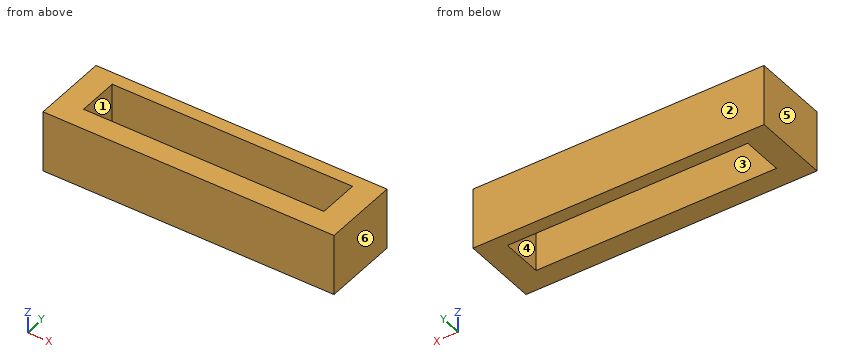
Autodesk Inventor part; units mm, degrees
ref_plane "YZ Plane" through (0, 0, 0) normal (1, 0, 0) x (0, 1, 0)
ref_plane "XZ Plane" through (0, 0, 0) normal (0, 1, 0) x (-1, 0, 0)
ref_plane "XY Plane" through (0, 0, 0) normal (0, 0, 1) x (1, 0, 0)
sketch "Sketch1" plane through (0, 0, 0) normal (0, 1, 0) x (-1, 0, 0)
  line L0 (-19.3909, 30.3636) -> (13.9091, 30.3636)
  line L1 (13.9091, 30.3636) -> (13.9091, 37.3636)
  line L2 (13.9091, 37.3636) -> (-19.3909, 37.3636)
  line L3 (-19.3909, 37.3636) -> (-19.3909, 30.3636)
  point P0 (0, 0)
  dimension "d0" = 33.3
  dimension "d1" = 7
extrude "MainBody" add sketch "Sketch1" along normal blind 2.5
sketch "Sketch2" plane through (0, 2.5, 0) normal (0, 1, 0) x (1, 0, 0)
  line L0 (-13.9091, -30.3636) -> (-13.9091, -37.3636)
  line L1 (-13.9091, -30.3636) -> (-11.0091, -30.3636)
  line L2 (-11.0091, -30.3636) -> (-11.0091, -37.3636)
  line L3 (-11.0091, -37.3636) -> (-13.9091, -37.3636)
  line L4 (-13.9091, -37.3636) -> (-13.9091, -30.3636)
  line L5 (-13.9091, -37.3636) -> (19.3909, -37.3636)
  line L6 (19.3909, -37.3636) -> (19.3909, -30.3636)
  line L7 (16.4909, -37.3636) -> (19.3909, -37.3636)
  line L8 (19.3909, -37.3636) -> (19.3909, -30.3636)
  line L9 (19.3909, -30.3636) -> (16.4909, -30.3636)
  line L10 (16.4909, -30.3636) -> (16.4909, -37.3636)
  line L11 (19.3909, -30.3636) -> (-13.9091, -30.3636)
  point P0 (0, 0)
  point P1 (-13.9091, -37.3636)
  dimension "ClipWidth" = 2.9
  dimension "d5" = 7
  dimension "d14" = 7
  dimension "d15" = 2.9
  dimension "d16" = 0
  dimension "d34" = 27.5
extrude "ClipHeight" add sketch "Sketch2" along normal blind 6.2 contours L1 L2 L3 L0 | L9 L6 L5 L10
sketch "Sketch4" plane through (-11.0091, 2.5, 37.3636) normal (1, 0, 0) x (0, 0, -1)
  line L0 (7, 0) -> (7, 6.2)
  line L1 (0, 0) -> (0, 6.2)
  line L2 (7, 6.2) -> (0, 6.2)
  line L3 (0, 6.2) -> (0, 4.7)
  line L4 (0, 4.7) -> (7, 4.7)
  line L5 (7, 4.7) -> (7, 6.2)
  line L6 (7, 6.2) -> (0, 6.2)
  point P0 (37.3636, -2.5)
  dimension "d9" = 1.5
extrude "Clip1_Out" add sketch "Sketch4" along normal blind 13.85
sketch "Sketch7" plane through (16.4909, 2.5, 30.3636) normal (-1, 0, 0) x (0, 0, 1)
  line L0 (0, 0) -> (0, 6.2)
  line L1 (7, 0) -> (7, 6.2)
  line L2 (0, 4.7) -> (7, 4.7)
  line L3 (7, 4.7) -> (7, 6.2)
  line L4 (7, 6.2) -> (0, 6.2)
  line L5 (0, 6.2) -> (0, 4.7)
  point P0 (-30.3636, -2.5)
  dimension "d22" = 1.5
  dimension "d23" = 7
extrude "Clip2_Out" add sketch "Sketch7" along normal blind 13.65
equation "\"d14\" = d5"
equation "\"d15\" = ClipWidth"
properties part number "Clip-on"
Check sheet for the modelled part. Datum: model origin and axes. Units: mm. Face numbers are marked on the shaded views. A direction names the side the tool comes from. Give positions to 0.01 mm unless a question says otherwise; leave off trailing zeros. Write each loop counter-clockwise with the first axis right and the second up, starting at its lowest first coordinate (ties: lowest second). Pieces come first, ordered by that corner, then holes. Notation, with made-up numbers: (-38, -25.5) -> (-27, -25.5) arc R7 cw to (-27, -16.5) -> close; hole circle Ø5 at (6, 8.25). An arc over 180 degrees is marked (long way). Use one line per item in the form item = value. Start each with the question number.
1. Go/stop test with a flat-tipped pin: P1, Ø2, axis at x = -7.5, y = 4.5, coming from the -Z side. Record where the tip stops, or that it passes through.
2. Section check C-C (z = 33.5). Record the cut outline in (x, y), and give its area (3 significant figures).
3. Thickness scan on line 1 along Y through (x, z) = (-7.5, 37.25); line 2 along X through (y, z) = (6.25, 31.5). Record the ranges inside material, lowest first. Write a range as from..to.
4. Section check A-A (y = 4). Record the cut outline in (x, z).
5. Access from +Z, -Z, +X, -X, +Y, -Y to the whole of each face (thin tool, end or side, straight path). Record for the marked faces 1 and 2.
6. Mould release check, pull along X, two halves, no side actions. Record for the marked faces 3, 4, 5 and 6: pulls with the +X half, pulls with the -X half, needs draft (parallel to the pull), parting line crosses it, or undercut.
7. Section check B-B (x = 12). Record the cut outline in (y, z).
Conclusion:
q1.P1 = through
q2.outline = (-13.91, 0) -> (19.39, 0) -> (19.39, 8.7) -> (-13.91, 8.7) -> close; hole (-11.01, 2.5) -> (16.49, 2.5) -> (16.49, 7.2) -> (-11.01, 7.2) -> close
q2.area = 160 mm²
q3.line_1 = 0..2.5, 7.2..8.7
q3.line_2 = -13.91..-11.01, 16.49..19.39
q4.outline = (-13.91, 30.36) -> (-11.01, 30.36) -> (-11.01, 37.36) -> (-13.91, 37.36) -> close; (16.49, 30.36) -> (19.39, 30.36) -> (19.39, 37.36) -> (16.49, 37.36) -> close
q5.face_1 = +Z, -Z
q5.face_2 = +Z, -Z, +X, -X, +Y
q6.face_3 = undercut
q6.face_4 = undercut
q6.face_5 = pulls with the -X half
q6.face_6 = pulls with the +X half
q7.outline = (0, 30.36) -> (2.5, 30.36) -> (2.5, 37.36) -> (0, 37.36) -> close; (7.2, 30.36) -> (8.7, 30.36) -> (8.7, 37.36) -> (7.2, 37.36) -> close
